from build123d import *

# Parameters (mm, degrees)
SKETCH1_W           = 25
SKETCH1_H           = 30
BOSS_EXTRUDE1_DEPTH = 7
SKETCH2_R           = 10
CUT_EXTRUDE1_DEPTH  = 3
FILLET1_R           = 10
FILLET2_R           = 10


with BuildPart() as part:
    # Sketch1 → Boss-Extrude1 (new body)
    with BuildSketch(Plane(origin=(0, 0, 0), x_dir=(1, 0, 0), z_dir=(0, 1, 0))):
        Rectangle(SKETCH1_W, SKETCH1_H)
    extrude(amount=BOSS_EXTRUDE1_DEPTH)

    # Sketch2 → Cut-Extrude1 (cut)
    with BuildSketch(Plane(origin=(0, 0, 0), x_dir=(1, 0, 0), z_dir=(0, 1, 0))):
        with Locations(Location((0, -3, 0), (0, 0, 270))):
            Circle(SKETCH2_R)
    extrude(amount=CUT_EXTRUDE1_DEPTH, mode=Mode.SUBTRACT)

    # Fillet1
    fillet1_edges = [part.edges().sort_by_distance(p)[0] for p in [
        (-12.5, 3.5, 15),
    ]]
    fillet(fillet1_edges, radius=FILLET1_R)

    # Fillet2
    fillet2_edges = [part.edges().sort_by_distance(p)[0] for p in [
        (12.5, 3.5, 15),
    ]]
    fillet(fillet2_edges, radius=FILLET2_R)


solid = part.part
Here's how the part is built. I have some questions about the finished solid (model axes, mm). Give positions to 0.01 mm unless a question says otherwise; leave off trailing zeros. Loops run counter-clockwise (first coordinate to the right, second up) from the corner with the lowest first, then second, coordinate; pieces in that order, holes last. Notation, with made-up numbers: (61.25, 12) -> (119.25, 12) arc R21 ccw to (119.25, 23) -> close; hole circle Ø10 at (41.5, -26). An arc over 180 degrees is marked (long way). Answer as a JSON object with one key per item and string values. Group by question number.
Item 1: Imagine slicing it at B-B on x = 0. Write out the boundary of the cut face in (y, z), then the cut area to 3 significant figures.
Item 2: Imagine slicing it at D-D on y = 5.5. Write out the boundary of the cut face in (x, z).
Item 3: Will these pins go through, and if not, where does the flat tip stop? pin 1 (1 mm diameter, centred on y = 4, z = 6, fed in from +X); pin 2 (10 mm diameter, centred on x = 0, z = 3.5, fed in from -Y).
Item 4: Thinking about a two-plate mould opening in Z: for faces 1 (the flat face through (0, 3, 15)), 2 (the cylindrical face through (3, 1.48, 12.54)), 3 (the flat face through (3, 0, -7)), 4 (the flat face through (0, 3, 3)), which applies, pulls with the +Z half, pulls with the -Z half, needs draft (parallel to the pull), parting line crosses it, or undercut?
Item 5: Imagine slicing it at A-A on y = 1.75. Write out the boundary of the cut face in (x, z).
Item 6: Imagine slicing it at C-C on z = 3. Write out the boundary of the cut face in (x, y), then the cut area to 3 significant figures.
Item 7: I need wall thicknesses on L1, parallel to X at y = 2.1, z = 3; L2, parallel to X at y = 1.25, z = 9; L3, parallel to Z at x = 0.75, y = 1. Which ranges of each line are inside material? Lowest first, please.
Answer list:
{
 "1": {"outline": "(0, -15) -> (7, -15) -> (7, 15) -> (0, 15) -> (0, 13) -> (3, 13) -> (3, -7) -> (0, -7) -> close", "area": "150 mm2"},
 "2": {"outline": "(-12.5, -15) -> (12.5, -15) -> (12.5, 5) arc R10 ccw to (2.5, 15) -> (-2.5, 15) arc R10 ccw to (-12.5, 5) -> close"},
 "3": {"pin 1": "stops at x = 12.49", "pin 2": "stops at y = 3"},
 "4": {"face 1": "pulls with the +Z half", "face 2": "undercut", "face 3": "needs draft", "face 4": "undercut"},
 "5": {"outline": "(-12.5, -15) -> (12.5, -15) -> (12.5, 5) arc R10 ccw to (2.5, 15) -> (-2.5, 15) arc R10 ccw to (-12.5, 5) -> close; hole circle Ø20 at (0, 3)"},
 "6": {"outline": "(-12.5, 0) -> (-10, 0) -> (-10, 3) -> (10, 3) -> (10, 0) -> (12.5, 0) -> (12.5, 7) -> (-12.5, 7) -> close", "area": "115 mm2"},
 "7": {"L1": "x = -12.5 to -10, 10 to 12.5", "L2": "x = -11.67 to -8, 8 to 11.67", "L3": "z = -15 to -6.97, 12.97 to 15"}
}
